from build123d import *

# Parameters (mm, degrees)
F0_W        = 457.2
F0_H        = 50.8
F1_DEPTH    = 9.525
F2_W        = 19.05
F2_H        = 19.05
F3_DEPTH    = 25.4
F4_W        = 6.35
F4_H        = 25.4
F5_DEPTH    = 12.7
F6_W        = 6.35
F6_H        = 25.4
F7_DEPTH    = 12.7
F8_T1_DEPTH = 142.2021954046


# Not quite as in the source:
# - a fillet or chamfer that OpenCascade refuses, or shapes differently, is made with other operations: its cross-section is extruded or revolved along the edge and cut away or added
# - a feature names something its author has since deleted; it is built from what else it names


with BuildPart() as f1:
    # F0 (on Front) → F1 (new body, symmetric)
    with BuildSketch(Plane.XZ):
        Rectangle(F0_W, F0_H)
    extrude(amount=F1_DEPTH, both=True)

    # F2 (on face) → F3 (cut, symmetric)
    with BuildSketch(Plane.XY.offset(25.4)):
        Rectangle(F2_W, F2_H)
    extrude(amount=F3_DEPTH, both=True, mode=Mode.SUBTRACT)

    # F4 (on face) → F5 (join, symmetric)
    with BuildSketch(Plane.YZ.offset(228.6)):
        Rectangle(F4_W, F4_H)
    extrude(amount=F5_DEPTH, both=True)

    # F6 (on face) → F7 (join, symmetric)
    with BuildSketch(Plane(origin=(-228.6, 0, 0), x_dir=(0, -1, 0), z_dir=(-1, 0, 0))):
        Rectangle(F6_W, F6_H)
    extrude(amount=F7_DEPTH, both=True)

    # F8: chamfer of 2.286 x 26.1290995641 on 2 edges, made by hand

    # F8_s2 → F8_t1 (cut)
    with BuildSketch(Plane.XZ.offset(-71.1010977023)):
        Polygon((-239.014, 12.7), (-241.3, -13.4290995641), (-241.3, 12.7), align=None)
        Polygon((239.014, 12.7), (241.3, -13.4290995641), (241.3, 12.7), align=None)
    extrude(amount=F8_T1_DEPTH, mode=Mode.SUBTRACT)


solid = f1.part
Input: part model. Units: mm. Frame: model coordinates. A direction names the side the tool comes from. Give positions to 0.01 mm unless a question says otherwise; leave off trailing zeros. Write each loop counter-clockwise with the first axis right and the second up, starting at its lowest first coordinate (ties: lowest second). Pieces come first, ordered by that corner, then holes. Notation, with made-up numbers: M 59,43 L 116,43 A25 cw 116,56 Z; hole C 17,25.5 d5. An arc over 180 degrees is marked long. Write item = value, one per line. Start each with the question number.
1) Cut plane B-B on y = 6.5. Return the cut outline in (x, z) (3 decimals).
2) Cut plane C-C on z = -20. Return the cut outline in (x, y) (3 decimals).
3) First-contact query: pin 1 Ø9.5 at (y, z) = (3, -1) entering from -X; pin 2 Ø9.5 at (y, z) = (2.5, 0.5) entering from +X; pin 3 Ø14 at (x, z) = (237.5, -6.5) entering from +Y (3 decimals); pin 4 Ø14 at (x, z) = (-233, 4.5) entering from +Y (3 decimals). Flat tips, straight axial feed; report the tip coordinate or a pass-through.
4) Material intervals for line 1 along X through (y, z) = (6.75, 21.5) (3 decimals); line 2 along X through (y, z) = (-2.5, -22.5); line 3 along X through (y, z) = (1.25, -4), sorted ascending. Write a range as [from, to].
5) Draft query along X for faces 4 (the flat face through (-235, 3.175, 0)), 5 (the flat face through (0, 0, 0)). Return one class per face: +X half, -X half, draft (parallel to the pull), parting line (faces both ways), or undercut.
6) Cut plane A-A on z = 4.5. Return the cut outline in (x, y) (3 decimals).
7) Reachability of faces 1 (the flat face through (235, -3.175, 0)), 2 (the flat face through (235, 3.175, 0)), 3 (the flat face through (-9.525, 0, 13)) from +Z, -Z, +X, -X, +Y, -Y: full face, straight path, thin tool, end or side. Return the list, or none.
Solved:
q1.outline = M -228.6,-25.4 L 228.6,-25.4 L 228.6,25.4 L 9.525,25.4 L 9.525,0 L -9.525,0 L -9.525,25.4 L -228.6,25.4 Z
q2.outline = M -228.6,-9.525 L 228.6,-9.525 L 228.6,9.525 L -228.6,9.525 Z
q3.pin_1 = -240.63
q3.pin_2 = 240.5
q3.pin_3 = 3.175
q3.pin_4 = 9.525
q4.line_1 = [-228.6, -9.525], [9.525, 228.6]
q4.line_2 = [-228.6, 228.6]
q4.line_3 = [-240.48, 240.48]
q5.face_4 = draft
q5.face_5 = undercut
q6.outline = M -239.731,-3.175 L -228.6,-3.175 L -228.6,-9.525 L -9.525,-9.525 L -9.525,9.525 L -228.6,9.525 L -228.6,3.175 L -239.731,3.175 Z; M 9.525,-9.525 L 228.6,-9.525 L 228.6,-3.175 L 239.731,-3.175 L 239.731,3.175 L 228.6,3.175 L 228.6,9.525 L 9.525,9.525 Z
q7.face_1 = +Z, -Z, +X, -Y
q7.face_2 = +Z, -Z, +X, +Y
q7.face_3 = +Z, +Y, -Y
